Source: CAD feature listing. Evaluate the final solid. Frame: model axes, mm. A direction names the side the tool comes from. Coordinates: 2 decimals unless noted, no trailing zeros. Write each loop counter-clockwise with the first axis right and the second up, starting at its lowest first coordinate (ties: lowest second). Pieces come first, ordered by that corner, then holes. Notation, with made-up numbers: M 29.25,-39.5 L 73.25,-39.5 A14 ccw 73.25,-28.5 Z; hole C 84,18.5 d5. An arc over 180 degrees is marked long. One line per item, written item: value. Start each with the question number.
Item 1: Set-up query: faces 1 (the cylindrical face through (-36.519, -35.183, 3.028)), 2 (the flat face through (0, 0, 7)), 3 (the flat face through (-1, 1, 15)). Return all of +Z, -Z, +X, -X, +Y, -Y with unobstructed straight access to the full face (end or side cutting, diameter ignored); none if empty.
Item 2: Pin query (flat end, axial travel): P1, Ø4, axis at x = -11.5, y = -40, coming from the +Z side; P2, Ø4.5, axis at x = 49, y = -8, coming from the +Z side; P3, Ø3.5, axis at x = -45.48, y = 20.77, coming from the +Z side; P4, Ø3, axis at y = -17.5, z = 5.5, coming from the +X side. Return the tip coordinate at first contact, or that it passes through.
Item 3: Cut plane D-D, the plane y = 50. Output: boundary loops of the cut face in (x, z).
Item 4: Cut plane A-A, the plane z = 12. Output: boundary loops of the cut face in (x, y), then the cut area to 3 significant figures.
Item 5: Ray query, L1, parallel to Y at x = 0, z = 13.7; L2, parallel to X at y = -49, z = -1.5; L3, parallel to Z at x = 6.5, y = 40. Return the intervals inside material, ascending. Write a range as from..to.
Item 6: Mould query, pull axis Y, two halves, no side actions, for faces 4 (the cylindrical face through (-29.78, 42.18, 3.03)), 5 (the flat face through (4, -40, 5)). Classes: released by +Y, released by -Y, zero draft, split by the parting line, or undercut.
Item 7: Cut plane B-B, the plane y = 0. Output: boundary loops of the cut face in (x, z), then the cut area to 3 significant figures.
Item 8: Cut plane C-C, the plane z = 2.5. State how many separate pieces and enclosed holes the cut face has, then the cut area to 3 significant figures.
```python
from build123d import *

# Parameters (mm, degrees)
SKETCH1_R           = 55
SKETCH1_R_2         = 1.5
BOSS_EXTRUDE1_DEPTH = 15
CUT_EXTRUDE2_START  = -10
SKETCH3_R           = 55
SKETCH3_R_2         = 17.5
CUT_EXTRUDE2_DEPTH  = 10
SKETCH7_R           = 12
CUT_EXTRUDE4_DEPTH  = 8
SKETCH8_R           = 37.5
BOSS_EXTRUDE2_DEPTH = 10
SKETCH9_R           = 12
CUT_EXTRUDE5_DEPTH  = 7
BOSS_EXTRUDE3_START = 3
SKETCH12_R          = 55
SKETCH12_R_2        = 12
SKETCH12_R_3        = 1.5
BOSS_EXTRUDE3_DEPTH = 3
SKETCH13_R          = 2.75
CUT_EXTRUDE7_DEPTH  = 4
SKETCH16_R          = 40
BOSS_EXTRUDE5_DEPTH = 10
SKETCH17_R          = 12
CUT_EXTRUDE8_DEPTH  = 2
SKETCH18_R          = 1.5
CUT_EXTRUDE9_DEPTH  = 5


with BuildPart() as part:
    # Sketch1 → Boss-Extrude1 (new body)
    with BuildSketch(Plane.XY):
        Circle(SKETCH1_R)
        with Locations((0, 50)):
            Circle(SKETCH1_R_2, mode=Mode.SUBTRACT)
        with Locations((27.032040873, 42.062676642)):
            Circle(SKETCH1_R_2, mode=Mode.SUBTRACT)
        with Locations((45.481599768, 20.77075065)):
            Circle(SKETCH1_R_2, mode=Mode.SUBTRACT)
        with Locations((49.491072094, -7.115741914)):
            Circle(SKETCH1_R_2, mode=Mode.SUBTRACT)
        with Locations((37.787478718, -32.743036697)):
            Circle(SKETCH1_R_2, mode=Mode.SUBTRACT)
        with Locations((14.086627842, -47.974648681)):
            Circle(SKETCH1_R_2, mode=Mode.SUBTRACT)
        with Locations((-14.086627842, -47.974648681)):
            Circle(SKETCH1_R_2, mode=Mode.SUBTRACT)
        with Locations((-37.787478718, -32.743036697)):
            Circle(SKETCH1_R_2, mode=Mode.SUBTRACT)
        with Locations((-49.491072094, -7.115741914)):
            Circle(SKETCH1_R_2, mode=Mode.SUBTRACT)
        with Locations((-45.481599768, 20.77075065)):
            Circle(SKETCH1_R_2, mode=Mode.SUBTRACT)
        with Locations((-27.032040873, 42.062676642)):
            Circle(SKETCH1_R_2, mode=Mode.SUBTRACT)
    extrude(amount=BOSS_EXTRUDE1_DEPTH)

    # Sketch3 → Cut-Extrude2 (cut)
    with BuildSketch(Plane.XY.offset(15).offset(CUT_EXTRUDE2_START)):
        Circle(SKETCH3_R)
        Circle(SKETCH3_R_2, mode=Mode.SUBTRACT)
    extrude(amount=CUT_EXTRUDE2_DEPTH, mode=Mode.SUBTRACT)

    # Sketch7 → Cut-Extrude4 (cut)
    with BuildSketch(Plane(origin=(0, 0, 0), x_dir=(-1, 0, 0), z_dir=(0, 0, -1))):
        Circle(SKETCH7_R)
    extrude(amount=-CUT_EXTRUDE4_DEPTH, mode=Mode.SUBTRACT)

    # Sketch8 → Boss-Extrude2 (add)
    with BuildSketch(Plane.XY.offset(5)):
        Circle(SKETCH8_R)
    extrude(amount=BOSS_EXTRUDE2_DEPTH)

    # Sketch9 → Cut-Extrude5 (cut)
    with BuildSketch(Plane(origin=(0, 0, 0), x_dir=(-1, 0, 0), z_dir=(0, 0, -1))):
        Circle(SKETCH9_R)
    extrude(amount=-CUT_EXTRUDE5_DEPTH, mode=Mode.SUBTRACT)

    # Sketch12 → Boss-Extrude3 (add)
    with BuildSketch(Plane(origin=(0, 0, 0), x_dir=(-1, 0, 0), z_dir=(0, 0, -1)).offset(BOSS_EXTRUDE3_START)):
        Circle(SKETCH12_R)
        Circle(SKETCH12_R_2, mode=Mode.SUBTRACT)
        with Locations((0, 50)):
            Circle(SKETCH12_R_3, mode=Mode.SUBTRACT)
        with Locations((27.032040873, 42.062676642)):
            Circle(SKETCH12_R_3, mode=Mode.SUBTRACT)
        with Locations((45.481599768, 20.77075065)):
            Circle(SKETCH12_R_3, mode=Mode.SUBTRACT)
        with Locations((49.491072094, -7.115741914)):
            Circle(SKETCH12_R_3, mode=Mode.SUBTRACT)
        with Locations((37.787478718, -32.743036697)):
            Circle(SKETCH12_R_3, mode=Mode.SUBTRACT)
        with Locations((14.086627842, -47.974648681)):
            Circle(SKETCH12_R_3, mode=Mode.SUBTRACT)
        with Locations((-14.086627842, -47.974648681)):
            Circle(SKETCH12_R_3, mode=Mode.SUBTRACT)
        with Locations((-37.787478718, -32.743036697)):
            Circle(SKETCH12_R_3, mode=Mode.SUBTRACT)
        with Locations((-49.491072094, -7.115741914)):
            Circle(SKETCH12_R_3, mode=Mode.SUBTRACT)
        with Locations((-45.481599768, 20.77075065)):
            Circle(SKETCH12_R_3, mode=Mode.SUBTRACT)
        with Locations((-27.032040873, 42.062676642)):
            Circle(SKETCH12_R_3, mode=Mode.SUBTRACT)
    extrude(amount=-BOSS_EXTRUDE3_DEPTH)

    # Sketch13 → Cut-Extrude7 (cut)
    with BuildSketch(Plane.XY.offset(5)):
        with Locations((0, 50)):
            Circle(SKETCH13_R)
        with Locations((27.032040873, 42.062676642)):
            Circle(SKETCH13_R)
        with Locations((45.481599768, 20.77075065)):
            Circle(SKETCH13_R)
        with Locations((49.491072094, -7.115741914)):
            Circle(SKETCH13_R)
        with Locations((37.787478718, -32.743036697)):
            Circle(SKETCH13_R)
        with Locations((14.086627842, -47.974648681)):
            Circle(SKETCH13_R)
        with Locations((-14.086627842, -47.974648681)):
            Circle(SKETCH13_R)
        with Locations((-37.787478718, -32.743036697)):
            Circle(SKETCH13_R)
        with Locations((-49.491072094, -7.115741914)):
            Circle(SKETCH13_R)
        with Locations((-45.481599768, 20.77075065)):
            Circle(SKETCH13_R)
        with Locations((-27.032040873, 42.062676642)):
            Circle(SKETCH13_R)
    extrude(amount=-CUT_EXTRUDE7_DEPTH, mode=Mode.SUBTRACT)

    # Sketch16 → Boss-Extrude5 (add)
    with BuildSketch(Plane.XY.offset(5)):
        Circle(SKETCH16_R)
    extrude(amount=BOSS_EXTRUDE5_DEPTH)

    # Sketch17 → Cut-Extrude8 (cut)
    with BuildSketch(Plane(origin=(0, 0, 5), x_dir=(-1, 0, 0), z_dir=(0, 0, -1))):
        Circle(SKETCH17_R)
    extrude(amount=-CUT_EXTRUDE8_DEPTH, mode=Mode.SUBTRACT)

    # Sketch18 → Cut-Extrude9 (cut)
    with BuildSketch(Plane.XY.offset(15)):
        with Locations((0, 20)):
            Circle(SKETCH18_R)
        with Locations((17.320508076, 10)):
            Circle(SKETCH18_R)
        with Locations((17.320508076, -10)):
            Circle(SKETCH18_R)
        with Locations((0, -20)):
            Circle(SKETCH18_R)
        with Locations((-17.320508076, -10)):
            Circle(SKETCH18_R)
        with Locations((-17.320508076, 10)):
            Circle(SKETCH18_R)
    extrude(amount=-CUT_EXTRUDE9_DEPTH, mode=Mode.SUBTRACT)


solid = part.part
```
From the geometry:
1. face 1: +Z
1. face 2: -Z
1. face 3: +Z, +X, -X, +Y, -Y
2. P1: stops at z = 15
2. P2: stops at z = 5
2. P3: stops at z = 1
2. P4: stops at x = 52.6
3. outline: M -22.91,-3 L -1.5,-3 L -1.5,1 L -2.75,1 L -2.75,5 L -22.91,5 Z; M 1.5,-3 L 22.91,-3 L 22.91,5 L 2.75,5 L 2.75,1 L 1.5,1 Z
4. outline: C 0,0 d80; hole C -17.32,-10 d3; hole C -17.32,10 d3; hole C 0,-20 d3; hole C 0,20 d3; hole C 17.32,-10 d3; hole C 17.32,10 d3
4. area: 4,980 mm²
5. L1: y = -40..-21.5, -18.5..18.5, 21.5..40
5. L2: x = -24.98..-15.18, -12.99..12.99, 15.18..24.98
5. L3: z = -3..5
6. face 4: undercut
6. face 5: zero draft
7. outline: M -55,-3 L -12,-3 L -12,7 L 12,7 L 12,-3 L 55,-3 L 55,5 L 40,5 L 40,15 L -40,15 L -40,5 L -55,5 Z
7. area: 1,440 mm²
8. separate pieces: 1
8. enclosed holes: 12
8. area: 8,790 mm²
